Model file for the job. Use its own axes, mm. Give positions to 0.01 mm unless a question says otherwise; leave off trailing zeros. Loops run counter-clockwise (first coordinate to the right, second up) from the corner with the lowest first, then second, coordinate; pieces in that order, holes last. Notation, with made-up numbers: M 51,-8 L 85,-8 A33 cw 85,22 Z; hole C 50,-18 d6. An arc over 180 degrees is marked long. Use CSV: the item, a comma, the result in double quotes. Start each with the question number.
(1) Flat gauge pin, fed straight in: P1, Ø1, axis at x = 3, y = 0.5, coming from the -Z side (3 decimals). Where does the tip first touch, or does it go through?
(2) Two-plate mould, pull along Z, no slides. Class faces 1 (the face through (13.67, 1.57, 3.03)), 2 (the face through (3, 0, 3)), 3 (the face through (-1.93, 1.61, -2.52)): pulls with the +Z half, pulls with the -Z half, needs draft (parallel to the pull), parting line crosses it, or undercut.
(3) Slice it at D-D on z = -9. List the corners of the cut face in (x, y) (3 decimals), and give its area (3 significant figures).
(4) Slice it at B-B on x = 0. List the corners of the cut face in (y, z) (3 decimals).
(5) Slice it at C-C on y = 2.3. List the corners of the cut face in (x, z) (3 decimals), and give its area (3 significant figures).
(6) Wall check: line 1 along Z through (x, y) = (1.25, 1.05); line 2 along X through (y, z) = (2.1, 0) (3 decimals); line 3 along X through (y, z) = (1.75, -9) (3 decimals). Give the ranges that are in metal, low to high. Write a range as from..to.
(7) Slice it at A-A on z = 0. List the corners of the cut face in (x, y) (3 decimals).
```python
from build123d import *

# Parameters (mm, degrees)
SKETCH1_R           = 14
BOSS_EXTRUDE1_DEPTH = 3.18
SKETCH2_R           = 3.175
CUT_EXTRUDE1_DEPTH  = 21.052740461
SKETCH3_R           = 3.175
CUT_EXTRUDE2_DEPTH  = 21.052740461


with BuildPart() as part:
    # Sketch1 → Boss-Extrude1 (new body)
    with BuildSketch(Plane(origin=(0, 0, 0), x_dir=(1, 0, 0), z_dir=(0, 1, 0))):
        with Locations(Location((0, 0, 0), (0, 0, 90))):
            Circle(SKETCH1_R)
    extrude(amount=BOSS_EXTRUDE1_DEPTH)

    # Sketch2 → Cut-Extrude1 (cut, through all)
    with BuildSketch(Plane(origin=(0, 3.18, 0), x_dir=(1, 0, 0), z_dir=(0, 1, 0))):
        with Locations(Location((0, 0, 0), (0, 0, 270))):
            Circle(SKETCH2_R)
    extrude(amount=-CUT_EXTRUDE1_DEPTH, mode=Mode.SUBTRACT)

    # Sketch3 → Cut-Extrude2 (cut, through all)
    with BuildSketch(Plane(origin=(0, 3.18, 0), x_dir=(1, 0, 0), z_dir=(0, 1, 0))):
        with Locations(Location((0, 9, 0), (0, 0, 270))):
            Circle(SKETCH3_R)
    extrude(amount=-CUT_EXTRUDE2_DEPTH, mode=Mode.SUBTRACT)


solid = part.part
```
Reply:
1,P1,"stops at z = -13.775"
2,face 1,"parting line crosses it"
2,face 2,"needs draft"
2,face 3,"undercut"
3,outline,"M -10.724,0 L -3.175,0 L -3.175,3.18 L -10.724,3.18 Z; M 3.175,0 L 10.724,0 L 10.724,3.18 L 3.175,3.18 Z"
3,area,"48.0 mm^2"
4,outline,"M 0,-14 L 3.18,-14 L 3.18,-12.175 L 0,-12.175 Z; M 0,-5.825 L 3.18,-5.825 L 3.18,-3.175 L 0,-3.175 Z; M 0,3.175 L 3.18,3.175 L 3.18,14 L 0,14 Z"
5,outline,"C 0,0 d28; hole C 0,-9 d6.35; hole C 0,0 d6.35"
5,area,"552 mm^2"
6,line 1,"z = -13.94..-11.92, -6.08..-2.92, 2.92..13.94"
6,line 2,"x = -14..-3.175, 3.175..14"
6,line 3,"x = -10.724..-3.175, 3.175..10.724"
7,outline,"M -14,0 L -3.175,0 L -3.175,3.18 L -14,3.18 Z; M 3.175,0 L 14,0 L 14,3.18 L 3.175,3.18 Z"
